Read the model definition and answer for the solid it produces. Units are mm, in the model's axes. Face numbers are marked on the shaded views. A direction names the side the tool comes from. Coordinates: 2 decimals unless noted, no trailing zeros. Order: outer loops, then holes, each group sorted by start corner. A loop starts at its lowest first (then second) coordinate and runs counter-clockwise, first axis right, second up.
Autodesk Inventor part; units mm, degrees
ref_plane "YZ Plane" through (0, 0, 0) normal (1, 0, 0) x (0, 1, 0)
ref_plane "XZ Plane" through (0, 0, 0) normal (0, 1, 0) x (-1, 0, 0)
ref_plane "XY Plane" through (0, 0, 0) normal (0, 0, 1) x (1, 0, 0)
sketch "Sketch5" plane through (0, 0, 0) normal (0, 0, 1) x (1, 0, 0)
  line L0 (-12.5, 6) -> (12.5, 6)
  line L1 (12.5, 6) -> (12.5, -6)
  line L2 (12.5, -6) -> (-12.5, -6)
  line L3 (-12.5, -6) -> (-12.5, 6)
  point P0 (0, 0)
  point P1 (0, 6)
  point P2 (12.5, 0)
  dimension "d8" = 25
  dimension "d9" = 12
extrude "Extrusion5" add sketch "Sketch5" along normal blind 9.5
sketch "Sketch6" plane through (0, 0, 9.5) normal (0, 0, 1) x (1, 0, 0)
  circle A0 centre (0, 0) radius 2
  dimension "d12" = 4
hole "Hole1" at (0, 0, 9.5) direction (0, 0, -1) diameter 4.2 end through all counterbore diameter 7.5 counterbore depth 4.5
chamfer "Chamfer2" distance 0.5 angle 45 4 edges at (0, -6, 9.5) (0, 6, 9.5) (0, -6, 0) (0, 6, 0)
chamfer "Chamfer3" distance 0.5 angle 45 4 edges at (12.5, 6, 4.75) (-12.5, 6, 4.75) (-12.5, -6, 4.75) (12.5, -6, 4.75)
chamfer "Chamfer4" distance 0.5 angle 45 1 edges at (0, 3.75, 9.5)
properties part number "BC-10025" material "Aço Inox AISI 304"
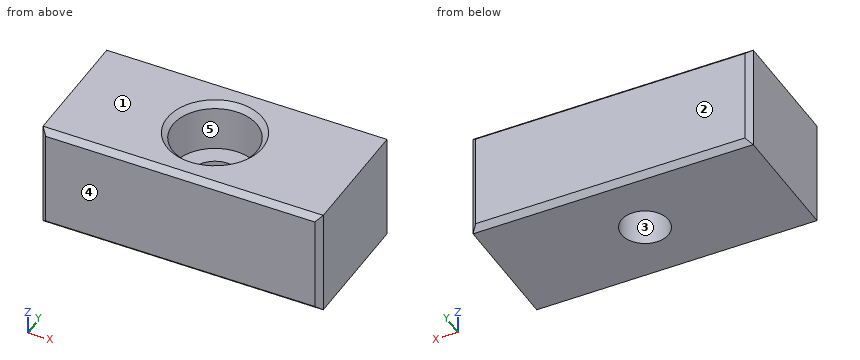
Q1. Which of the six approach directions +Z, -Z, +X, -X, +Y, -Y give full straight-line access (tool end or side, diameter ignored) to the marked faces 4 and 5?
Q2. Straight lines are drawn through the part: L1, parallel to Y at x = 0, z = 2.35; L2, parallel to Y at x = 0, z = 7.3; L3, parallel to X at y = 0, z = 8. For each, find the intervals that lie inside material, in ascending order.
Q3. Determine the mould class of the marked faces 1, 2 and 3 for opening direction Y: +Y half, -Y half, draft (parallel to the pull), parting line (faces both ways), or undercut.
Q4. The part is cut by section C-C, the plane y = 0. Determine the outline of the cut face in (x, z).
Q5. The part is cut by section D-D, the plane z = 7. Determine the outline of the cut face in (x, y), then the cut area to 3 significant figures.
Q6. The part is cut by section A-A, the plane z = 3. Determine the outline of the cut face in (x, y), then the cut area to 3 significant figures.
Q7. The part is cut by section B-B, the plane x = 0. Determine the outline of the cut face in (y, z).
Q8. This flat-tipped pin is pushed along its axis until it touches: P1, Ø6, axis at x = -0.5, y = 0.5, coming from the +Z side. Where does it stop, or does it pass through?
Computed values:
1. face 4: +Z, -Z, +X, -X, -Y
1. face 5: +Z
2. L1: y = -6 to -2.1, 2.1 to 6
2. L2: y = -6 to -3.75, 3.75 to 6
2. L3: x = -12.5 to -3.75, 3.75 to 12.5
3. face 1: draft
3. face 2: +Y half
3. face 3: undercut
4. outline: (-12.5, 0) - (-2.1, 0) - (-2.1, 5) - (-3.75, 5) - (-3.75, 9) - (-4.25, 9.5) - (-12.5, 9.5) - close; (2.1, 0) - (12.5, 0) - (12.5, 9.5) - (4.25, 9.5) - (3.75, 9) - (3.75, 5) - (2.1, 5) - close
5. outline: (-12.5, -5.5) - (-12, -6) - (12, -6) - (12.5, -5.5) - (12.5, 5.5) - (12, 6) - (-12, 6) - (-12.5, 5.5) - close; hole circle Ø7.5 at (0, 0)
5. area: 255 mm2
6. outline: (-12.5, -5.5) - (-12, -6) - (12, -6) - (12.5, -5.5) - (12.5, 5.5) - (12, 6) - (-12, 6) - (-12.5, 5.5) - close; hole circle Ø4.2 at (0, 0)
6. area: 286 mm2
7. outline: (-6, 0.5) - (-5.5, 0) - (-2.1, 0) - (-2.1, 5) - (-3.75, 5) - (-3.75, 9) - (-4.25, 9.5) - (-5.5, 9.5) - (-6, 9) - close; (2.1, 0) - (5.5, 0) - (6, 0.5) - (6, 9) - (5.5, 9.5) - (4.25, 9.5) - (3.75, 9) - (3.75, 5) - (2.1, 5) - close
8. P1: stops at z = 5
